from build123d import *
from build123d.topology import SkipClean

# Parameters (mm, degrees)
BOSS_EXTRUDE3_DEPTH   = 8
SKETCH2_R             = 4.5
BOSS_EXTRUDE3_2_DEPTH = 8
SKETCH4_W             = 25.128147065
SKETCH4_H             = 19.783027293
BOSS_EXTRUDE4_DEPTH   = 3
SKETCH5_W             = 19.783027293
SKETCH5_H             = 11
BOSS_EXTRUDE5_DEPTH   = 3
BOSS_EXTRUDE6_START   = -8
BOSS_EXTRUDE6_DEPTH   = 8


with BuildPart() as part:
    # Sketch2 → Boss-Extrude3 (new body)
    with BuildSketch(Plane(origin=(0, 0, 0), x_dir=(1, 0, 0), z_dir=(0, 1, 0))):
        with BuildLine():
            Line((0, 19.783027293), (0, 11.408726598))
            Line((0, 11.408726598), (9.090512027, 11.408726598))
            ThreePointArc((9.090512027, 11.408726598), (10.598731266, 11.815413134), (11.698035534, 12.925210115))
            ThreePointArc((11.698035534, 12.925210115), (23.1, 9.908726598), (11.698035534, 6.892243082))
            ThreePointArc((11.698035534, 6.892243082), (10.598731266, 8.002040063), (9.090512027, 8.408726598))
            Line((9.090512027, 8.408726598), (0, 8.408726598))
            Line((0, 8.408726598), (0, 0))
            Line((0, 0), (25.128147065, 0))
            Line((25.128147065, 0), (25.128147065, 19.783027293))
            Line((25.128147065, 19.783027293), (0, 19.783027293))
        make_face()
    extrude(amount=BOSS_EXTRUDE3_DEPTH)



with BuildPart() as body_2:
    # Sketch2 → Boss-Extrude3 2 (new body)
    with BuildSketch(Plane(origin=(0, 0, 0), x_dir=(1, 0, 0), z_dir=(0, 1, 0))):
        with Locations(Location((17, 9.908726598, 0), (0, 0, 270))):
            Circle(SKETCH2_R)
    extrude(amount=BOSS_EXTRUDE3_2_DEPTH)


with BuildPart() as part_1:
    add(part.part)

    add(body_2.part)  # Boss-Extrude4 merges body 2
    # Sketch4 → Boss-Extrude4 (add)
    with BuildSketch(Plane.XZ):
        with Locations((12.564073533, -9.891513646)):
            Rectangle(SKETCH4_W, SKETCH4_H)
    extrude(amount=BOSS_EXTRUDE4_DEPTH)

    # Sketch5 → Boss-Extrude5 (add)
    with BuildSketch(Plane(origin=(25.128147065, 0, 0), x_dir=(0, 0, -1), z_dir=(1, 0, 0))):
        with Locations((9.891513646, 2.5)):
            Rectangle(SKETCH5_W, SKETCH5_H)
    extrude(amount=BOSS_EXTRUDE5_DEPTH)

    # Sketch6 → Boss-Extrude6 (add)
    with SkipClean():  # the faces are left unmerged after this step: merging them gives an invalid solid
        with BuildSketch(Plane(origin=(0, 8, 0), x_dir=(1, 0, 0), z_dir=(0, 1, 0)).offset(BOSS_EXTRUDE6_START)):
            with BuildLine():
                ThreePointArc((11.493419665, 12.533145203), (10.570986936, 11.494612896), (9.236624446, 11.108726598))
                Line((9.236624446, 11.108726598), (0, 11.108726598))
                Line((0, 11.108726598), (0, 11.408726598))
                Line((0, 11.408726598), (9.090512027, 11.408726598))
                ThreePointArc((9.090512027, 11.408726598), (10.598731266, 11.815413134), (11.698035534, 12.925210115))
                ThreePointArc((11.698035534, 12.925210115), (11.592173366, 12.731032588), (11.493419665, 12.533145203))
            make_face()
            with BuildLine():
                ThreePointArc((11.493419665, 7.284307994), (11.592173366, 7.086420609), (11.698035534, 6.892243082))
                ThreePointArc((11.698035534, 6.892243082), (10.598731266, 8.002040063), (9.090512027, 8.408726598))
                Line((9.090512027, 8.408726598), (0, 8.408726598))
                Line((0, 8.408726598), (0, 8.708726598))
                Line((0, 8.708726598), (9.236624446, 8.708726598))
                ThreePointArc((9.236624446, 8.708726598), (10.570986936, 8.3228403), (11.493419665, 7.284307994))
            make_face()
        extrude(amount=BOSS_EXTRUDE6_DEPTH)


solid = part_1.part
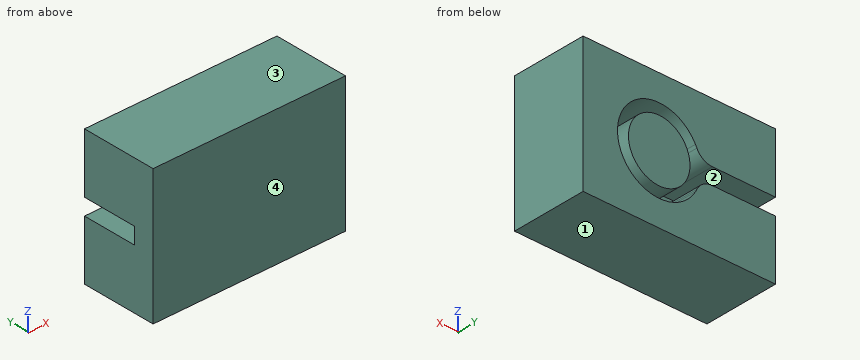
Can you work these out from the model? Positions are in its coordinate system, mm. Face numbers are marked on the shaded views. Coordinates: 2 decimals unless noted, no trailing zeros. Write each loop counter-clockwise with the first axis right and the second up, starting at its lowest first coordinate (ties: lowest second). Pieces come first, ordered by that corner, then holes. Notation, with made-up numbers: (25.25, 41) - (56.25, 41) arc R11 ccw to (56.25, 58) - close; hole circle Ø10 at (42.25, 8.5). An arc over 180 degrees is marked (long way). Return JSON: item names as keys, results as strings. Group by question number.
Item 1: If we section it at B-B (x = 17): Write out the boundary of the cut face in (y, z), then the cut area to 3 significant figures.
Item 2: If we section it at C-C (z = -12): Write out the boundary of the cut face in (x, y), then the cut area to 3 significant figures.
Item 3: Please list where these lines run through material, in increasing order: probe 1 along Z at (x, y) = (6.5, 1); probe 2 along Z at (x, y) = (14, 6.25); probe 3 along X at (y, z) = (2.75, -7.25).
Item 4: We'd pull the mould along Z, two halves only. Please class the marked faces 1, 2, 3 and 4: pulls with the +Z half, pulls with the -Z half, needs draft (parallel to the pull), parting line crosses it, or undercut.
Item 5: If we section it at D-D (x = 7): Write out the boundary of the cut face in (y, z), then the cut area to 3 significant figures.
Item 6: If we section it at A-A (y = 3.75): Write out the boundary of the cut face in (x, z), then the cut area to 3 significant figures.
Return value:
{
 "1": {"outline": "(-3, -19.78) - (8, -19.78) - (8, -16.01) - (0, -16.01) - (0, -14.41) - (8, -14.41) - (8, -5.41) - (0, -5.41) - (0, -3.81) - (8, -3.81) - (8, 0) - (-3, 0) - close", "area": "192 mm^2"},
 "2": {"outline": "(0, -3) - (28.13, -3) - (28.13, 8) - (22.73, 8) - (22.73, 0) - (20.98, 0) - (20.98, 8) - (13.02, 8) - (13.02, 0) - (11.15, 0) - (11.15, 8) - (0, 8) - close", "area": "281 mm^2"},
 "3": {"probe 1": "z = -19.78 to -11.11, -8.71 to 0", "probe 2": "z = -19.78 to -15.22, -13.26 to -6.55, -4.6 to 0", "probe 3": "x = 0 to 11.51, 13.37 to 20.63, 22.49 to 28.13"},
 "4": {"face 1": "pulls with the -Z half", "face 2": "undercut", "face 3": "pulls with the +Z half", "face 4": "needs draft"},
 "5": {"outline": "(-3, -19.78) - (8, -19.78) - (8, -11.11) - (0, -11.11) - (0, -8.71) - (8, -8.71) - (8, 0) - (-3, 0) - close", "area": "198 mm^2"},
 "6": {"outline": "(0, -19.78) - (28.13, -19.78) - (28.13, 0) - (0, 0) - (0, -8.71) - (9.24, -8.71) arc R2.5 ccw to (11.49, -7.28) arc R6.1 cw (long way) to (11.49, -12.53) arc R2.5 ccw to (9.24, -11.11) - (0, -11.11) - close; circle Ø9 at (17, -9.91)", "area": "476 mm^2"}
}
